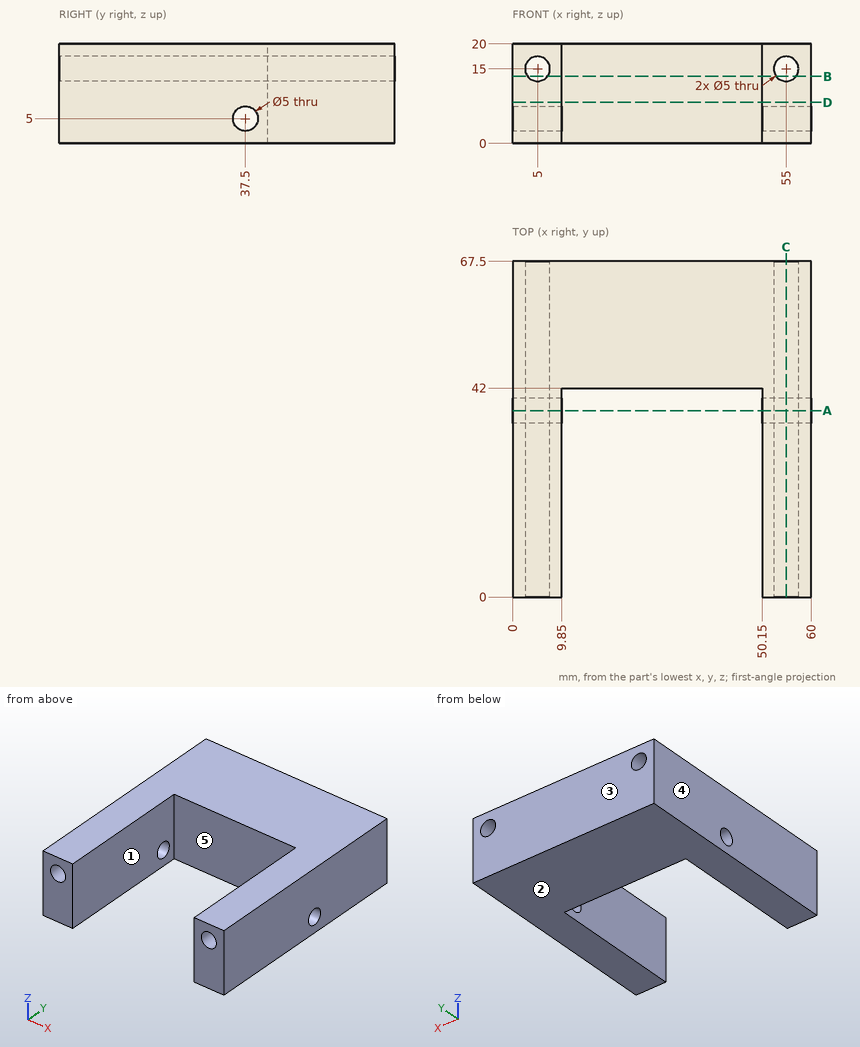
Answer from the drawing. Dimensions are ordinates in mm from the lowest x, y and z of the part. A direction names the side the tool comes from. Round coordinates to 2 decimals unless told otherwise and drop trailing zeros. Loops run counter-clockwise (first coordinate to the right, second up) from the corner with the lowest first, then second, coordinate; pieces in that order, holes last. Notation, with made-up numbers: M 82,-17.5 L 87,-17.5 A18 cw 87,7.5 Z; hole C 88,64 d8. An arc over 180 degrees is marked long. One line per question, with ' | ' between items. Start each with the question number.
(1) For a pull along X with two mould halves and no side action, classify the marked faces 3, 4 and 5 as released by +X, released by -X, zero draft, split by the parting line, or undercut.
(2) Flat-ended cylindrical pins translate along their axes: pin 1 Ø6 at (x, z) = (18, 4.5) entering from -Y; pin 2 Ø4.5 at (y, z) = (37.5, 5) entering from +X. Find the tip coordinate at first contact, or state that the pin passes through.
(3) A cutting plane is placed at D-D on z = 8.25. Write down the section's boundary in (x, y), plus the area to 3 significant figures.
(4) A tool of negligible diameter and unlimited length cuts with its end or side. For the marked faces 1 and 2, from which of +Z, -Z, +X, -X, +Y, -Y can it reach the whole face along a straight path? Write none if from no direction.
(5) A cutting plane is placed at C-C on x = 55. Write down the section's boundary in (y, z).
(6) Find the intervals of material crossed by line 1 (Z direction, x = 3, y = 37); line 2 (Z direction, x = 5, y = 20); line 3 (X direction, y = 19.5, z = 15.75), in increasing order.
(7) A cutting plane is placed at A-A on y = 37.5. Write down the section's boundary in (x, z).
(8) A cutting plane is placed at B-B on z = 13.5. Write down the section's boundary in (x, y).
Geometry check:
1) face 3: zero draft | face 4: released by -X | face 5: undercut
2) pin 1: stops at y = 42 | pin 2: passes through
3) outline: M 0,0 L 9.85,0 L 9.85,42 L 50.15,42 L 50.15,0 L 60,0 L 60,67.5 L 0,67.5 Z | area: 2,360 mm²
4) face 1: +Z, -Z, -Y | face 2: -Z, +X, -X, +Y, -Y
5) outline: M 0,0 L 67.5,0 L 67.5,12.5 L 0,12.5 Z; M 0,17.5 L 67.5,17.5 L 67.5,20 L 0,20 Z; hole C 37.5,5 d5
6) line 1: z = 0 to 2.55, 7.45 to 13.5, 16.5 to 20 | line 2: z = 0 to 12.5, 17.5 to 20 | line 3: x = 0 to 2.62, 7.38 to 9.85, 50.15 to 52.62, 57.38 to 60
7) outline: M 0,0 L 9.85,0 L 9.85,2.5 L 0,2.5 Z; M 0,7.5 L 9.85,7.5 L 9.85,20 L 0,20 Z; M 50.15,0 L 60,0 L 60,2.5 L 50.15,2.5 Z; M 50.15,7.5 L 60,7.5 L 60,20 L 50.15,20 Z; hole C 5,15 d5; hole C 55,15 d5
8) outline: M 0,0 L 3,0 L 3,67.5 L 0,67.5 Z; M 7,0 L 9.85,0 L 9.85,42 L 50.15,42 L 50.15,0 L 53,0 L 53,67.5 L 7,67.5 Z; M 57,0 L 60,0 L 60,67.5 L 57,67.5 Z
